For this review, take the finished solid that the model builds, in its own axes (mm). A direction names the side the tool comes from. Round coordinates to 2 decimals unless told otherwise and drop trailing zeros. Order: outer loops, then holes, each group sorted by start corner. A loop starts at its lowest first (then second) coordinate and runs counter-clockwise, first axis right, second up. Notation, with made-up numbers: (13.25, 83.5) - (43.25, 83.5) arc R27 cw to (43.25, 118.5) - close; hole circle Ø6 at (-21, 24.5). An arc over 180 degrees is marked (long way). Write each question's results on one line, items separated by ' | '. Start each with the question number.
(1) Take a section at A-A, the plane z = 50.5. Give the boundary of the cut face in (x, y).
(2) For faces 5 (the flat face through (13, 1.587, 157)), 6 (the cylindrical face through (24.617, 12.588, 143.512)), 7 (the cylindrical face through (15.22, 0.78, 14.62)), list the 3-axis set-ups (+Z, -Z, +X, -X, +Y, -Y) from which the entire face can be reached by the end or side of a thin tool; tool diameter is ignored.
(3) Draft analysis for pull direction X (two halves, no side actions). For faces 1 (the cylindrical face through (0.805, 12.812, 307.338)), 2 (the flat face through (0, 13, 157)), 3 (the flat face through (23.812, 13, 157)), 4 (the flat face through (13, 23.812, 157)), state which applies: pulls with the +X half, pulls with the -X half, needs draft (parallel to the pull), parting line crosses it, or undercut.
(4) For L1, parallel to Z at x = 12.25, y = 1.5; L2, parallel to Y at x = 21.25, z = 20, list the stretches that pass through material, from the lowest coordinate up. Write a range as from..to.
(5) Take a section at B-B, the plane y = 20.5. Give the boundary of the cut face in (x, z), plus the area to 3 significant figures.
(6) Insertion check: pin 1 Ø3 at (y, z) = (12.7, 146.05) entering from -X; pin 2 Ø3 at (x, z) = (12.7, 303.21) entering from -Y. Each pin has a flat end and moves straight along its axis. Give the tip position at first contact, or say it passes through.
```python
from build123d import *

# Parameters (mm, degrees)
SKETCH1_W           = 25.4
SKETCH1_H           = 25.4
SKETCH1_W_2         = 22.225
SKETCH1_H_2         = 22.225
BOSS_EXTRUDE1_DEPTH = 317.5
SKETCH4_R           = 2.54
CUT_EXTRUDE3_DEPTH  = 320.525538885
CUT_EXTRUDE4_REACH  = 321.526
SKETCH5_R           = 2.54


with BuildPart() as part:
    # Sketch1 → Boss-Extrude1 (new body)
    with BuildSketch(Plane.XY):
        with Locations((12.7, 12.7)):
            Rectangle(SKETCH1_W, SKETCH1_H)
        with Locations((12.7, 12.7)):
            Rectangle(SKETCH1_W_2, SKETCH1_H_2, mode=Mode.SUBTRACT)
    extrude(amount=BOSS_EXTRUDE1_DEPTH)

    # Sketch4 → Cut-Extrude3 (cut, through all)
    with BuildSketch(Plane(origin=(25.4, 0, 0), x_dir=(0, 0, -1), z_dir=(1, 0, 0))):
        with Locations((-304.8, 12.7)):
            Circle(SKETCH4_R)
        with Locations((-279.4, 12.7)):
            Circle(SKETCH4_R)
        with Locations(Location((-38.1, 12.7, 0), (0, 0, 180))):
            Circle(SKETCH4_R)
        with Locations(Location((-12.7, 12.7, 0), (0, 0, 180))):
            Circle(SKETCH4_R)
        with Locations((-171.45, 12.7)):
            Circle(SKETCH4_R)
        with Locations(Location((-146.05, 12.7, 0), (0, 0, 180))):
            Circle(SKETCH4_R)
    extrude(amount=-CUT_EXTRUDE3_DEPTH, mode=Mode.SUBTRACT)

    # Sketch5 → Cut-Extrude4 (cut, up to next)
    with BuildSketch(Plane.XZ, mode=Mode.PRIVATE) as cut_extrude4_sk1:
        with Locations(Location((12.7, 303.2125, 0), (0, 0, 270))):
            Circle(SKETCH5_R)
    cut_extrude4_tool1 = extrude(cut_extrude4_sk1.sketch, amount=-CUT_EXTRUDE4_REACH, mode=Mode.PRIVATE) & part.part
    # Sketch5 → Cut-Extrude4 (cut, up to next)
    with BuildSketch(Plane.XZ, mode=Mode.PRIVATE) as cut_extrude4_sk2:
        with Locations(Location((12.7, 14.2875, 0), (0, 0, 270))):
            Circle(SKETCH5_R)
    cut_extrude4_tool2 = extrude(cut_extrude4_sk2.sketch, amount=-CUT_EXTRUDE4_REACH, mode=Mode.PRIVATE) & part.part
    add(cut_extrude4_tool1.solids().sort_by_distance((12.7, 0, 303.2125))[0], mode=Mode.SUBTRACT)
    add(cut_extrude4_tool2.solids().sort_by_distance((12.7, 0, 14.2875))[0], mode=Mode.SUBTRACT)


solid = part.part
```
Results below:
1) outline: (0, 0) - (25.4, 0) - (25.4, 25.4) - (0, 25.4) - close; hole (1.59, 1.59) - (23.81, 1.59) - (23.81, 23.81) - (1.59, 23.81) - close
2) face 5: +Z, -Z | face 6: +X, -X | face 7: -Y
3) face 1: needs draft | face 2: pulls with the -X half | face 3: undercut | face 4: undercut
4) L1: z = 0..11.79, 16.79..300.71, 305.71..317.5 | L2: y = 0..1.59, 23.81..25.4
5) outline: (0, 0) - (1.59, 0) - (1.59, 317.5) - (0, 317.5) - close; (23.81, 0) - (25.4, 0) - (25.4, 317.5) - (23.81, 317.5) - close | area: 1,010 mm^2
6) pin 1: passes through | pin 2: stops at y = 23.81
